For this review, use the dimensioned drawing (mm, ordinates from the lowest corner) and the shaded views. Coordinates: 2 decimals unless noted, no trailing zeros. Loops run counter-clockwise (first coordinate to the right, second up) from the corner with the lowest first, then second, coordinate; pieces in that order, holes last. Notation, with made-up numbers: (38.25, 82.25) - (50.25, 82.25) arc R13 ccw to (50.25, 88.25) - close; hole circle Ø7 at (-1, -34). An arc over 180 degrees is marked (long way). Answer in a Markdown table with one row per item. Add a question column.
(1) Clearance check with a flat-ended pin moving along its axis: pin 1 (4 mm diameter, centred on x = 410, z = 4, fed in from -Y). State where the tip first meets the part, or that it passes through.
(2) We need section B-B, the plane z = 9.75. Write out the cut boundary in (x, y), plus the area to 3 significant figures.
(3) We need section C-C, the plane x = 1219.75. Write out the cut boundary in (y, z) (1 decimal), plus the area to 3 significant figures.
(4) We need section A-A, the plane y = 203.2. Write out the cut boundary in (x, z).
(5) To check wall thickness, follow L1, parallel to Y at x = 1219.75, z = 9.25 (1 decimal); L2, parallel to Y at x = 1222, z = 10; L3, parallel to Y at x = 1000.5, z = 4.75. State the ranges of each line that lie inside material, in increasing order. Write a range as [from, to].
(6) We need section D-D, the plane y = 452. Write out the cut boundary in (x, z), plus the area to 3 significant figures.
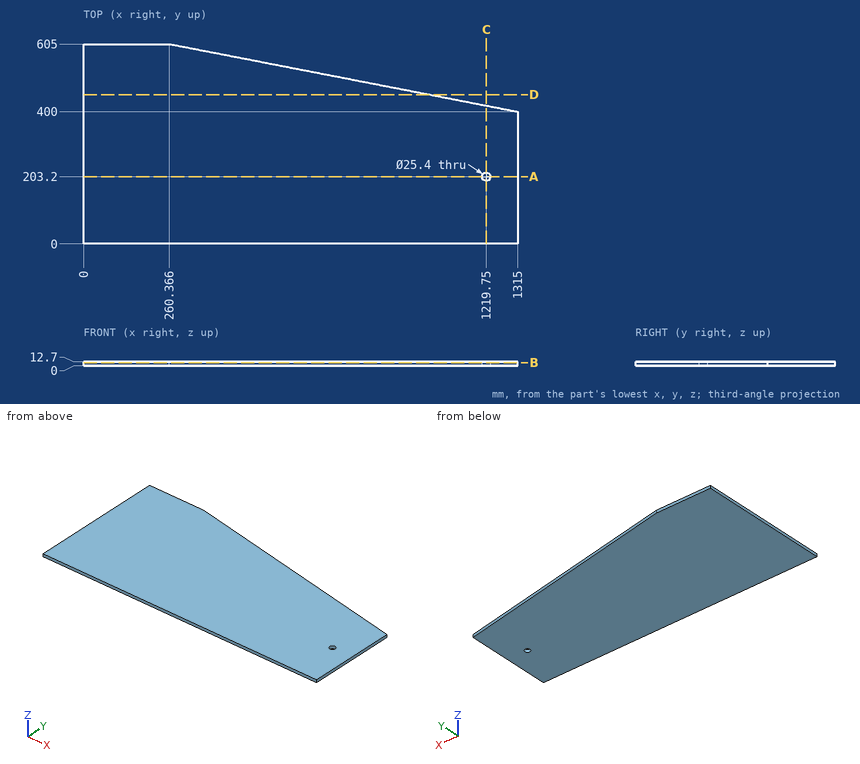
Responses:
| question | item | result |
|---|---|---|
| 1 | pin 1 | stops at y = 0 |
| 2 | outline | (0, 0) - (1315, 0) - (1315, 400) - (260.37, 605) - (0, 605) - close; hole circle Ø25.4 at (1219.75, 203.2) |
| 2 | area | 687,000 mm2 |
| 3 | outline | (0, 0) - (190.5, 0) - (190.5, 12.7) - (0, 12.7) - close; (215.9, 0) - (418.5, 0) - (418.5, 12.7) - (215.9, 12.7) - close |
| 3 | area | 4,990 mm2 |
| 4 | outline | (0, 0) - (1207.05, 0) - (1207.05, 12.7) - (0, 12.7) - close; (1232.45, 0) - (1315, 0) - (1315, 12.7) - (1232.45, 12.7) - close |
| 5 | L1 | y = [0, 190.5], [215.9, 418.5] |
| 5 | L2 | y = [0, 190.7], [215.7, 418.08] |
| 5 | L3 | y = [0, 461.13] |
| 6 | outline | (0, 0) - (1047.48, 0) - (1047.48, 12.7) - (0, 12.7) - close |
| 6 | area | 13,300 mm2 |
